Geometry: final body of the model. Coordinates: model frame, mm. Round coordinates to 2 decimals unless told otherwise and drop trailing zeros. Write each loop counter-clockwise with the first axis right and the second up, starting at its lowest first coordinate (ties: lowest second). Pieces come first, ordered by that corner, then holes. Notation, with made-up numbers: M 63,58.25 L 81,58.25 A13 ccw 81,78.25 Z; hole C 51.5,-39 d5. An arc over 180 degrees is marked long. Answer as CSV lines item,"result". Start each with the question number.
Q1. Section query C-C on y = 3. Output: boundary loops of the cut face in (x, z).
Q2. Ray query, probe 1 along X at (y, z) = (0.85, 22.5); probe 2 along Z at (x, y) = (-14, 3.5); probe 3 along Z at (x, y) = (-14, 1). Return the intervals inside material, ascending.
Q3. First-contact query: pin 1 (1 mm diameter, centred on y = 0.5, z = 13.5, fed in from -X); pin 2 (1.5 mm diameter, centred on x = -42, y = 1, fed in from +Z); pin 3 (2 mm diameter, centred on y = 1, z = 15, fed in from +X). Flat tips, straight axial feed; report the tip coordinate or a pass-through.
```python
from build123d import *

# Parameters (mm, degrees)
SKETCH1_W           = 200
SKETCH1_H           = 80
BOSS_EXTRUDE1_DEPTH = 2
SKETCH2_W           = 196
SKETCH2_H           = 76
BOSS_EXTRUDE2_DEPTH = 2
FILLET1_R           = 2
FILLET2_R           = 2
FILLET3_R           = 2
SKETCH3_R           = 33.072163117
CUT_EXTRUDE1_DEPTH  = 25
FILLET4_R           = 2
FILLET5_R           = 2
SKETCH4_W           = 18.581197799
SKETCH4_H           = 6.58
CUT_EXTRUDE3_DEPTH  = 2
SKETCH5_W           = 3.741738876
SKETCH5_H           = 6.58
CUT_EXTRUDE4_DEPTH  = 2
FILLET6_R           = 2
FILLET7_R           = 2


with BuildPart() as part:
    # Sketch1 → Boss-Extrude1 (new body)
    with BuildSketch(Plane(origin=(0, 0, 0), x_dir=(1, 0, 0), z_dir=(0, 1, 0))):
        Rectangle(SKETCH1_W, SKETCH1_H)
    extrude(amount=BOSS_EXTRUDE1_DEPTH)

    # Sketch2 → Boss-Extrude2 (add)
    with BuildSketch(Plane(origin=(0, 2, 0), x_dir=(1, 0, 0), z_dir=(0, 1, 0))):
        Rectangle(SKETCH2_W, SKETCH2_H)
    extrude(amount=BOSS_EXTRUDE2_DEPTH)

    # Fillet1
    fillet1_edges = [part.edges().sort_by_distance(p)[0] for p in [
        (-100, 1, -40),
        (100, 1, -40),
        (100, 1, 40),
        (-100, 1, 40),
    ]]
    fillet(fillet1_edges, radius=FILLET1_R)

    # Fillet2
    fillet2_edges = [part.edges().sort_by_distance(p)[0] for p in [
        (-98, 3, -38),
        (-98, 3, 38),
        (98, 3, 38),
        (98, 3, -38),
    ]]
    fillet(fillet2_edges, radius=FILLET2_R)

    # Fillet3
    fillet3_edges = [part.edges().sort_by_distance(p)[0] for p in [
        (-99.414213562, 0, -39.414213562),
        (0, 0, -40),
        (99.414213562, 0, -39.414213562),
        (100, 0, 0),
        (99.414213562, 0, 39.414213562),
        (0, 0, 40),
        (-99.414213562, 0, 39.414213562),
        (-97.414213562, 2, 37.414213562),
        (-98, 2, 0),
        (-97.414213562, 2, -37.414213562),
        (0, 2, -38),
        (97.414213562, 2, -37.414213562),
        (98, 2, 0),
        (97.414213562, 2, 37.414213562),
        (-100, 0, 0),
        (0, 2, 38),
    ]]
    fillet(fillet3_edges, radius=FILLET3_R - 0.0001)  # a hair under: the kernel refuses the full size

    # Sketch3 → Cut-Extrude1 (cut)
    with BuildSketch(Plane.XZ):
        with Locations(Location((-43.56, 0, 0), (0, 0, 270))):
            Circle(SKETCH3_R)
    extrude(amount=-CUT_EXTRUDE1_DEPTH, mode=Mode.SUBTRACT)

    # Fillet4
    fillet4_edges = [part.edges().sort_by_distance(p)[0] for p in [
        (-43.56, 0, 33.072163117),
    ]]
    fillet(fillet4_edges, radius=FILLET4_R)

    # Fillet5
    fillet5_edges = [part.edges().sort_by_distance(p)[0] for p in [
        (-43.56, 4, 33.072163117),
    ]]
    fillet(fillet5_edges, radius=FILLET5_R - 0.0001)  # a hair under: the kernel refuses the full size

    # Sketch4 → Cut-Extrude3 (cut)
    with BuildSketch(Plane(origin=(0, 4, 0), x_dir=(1, 0, 0), z_dir=(0, 1, 0))):
        with Locations((88.709401101, 20.450898194)):
            Rectangle(SKETCH4_W, SKETCH4_H)
    extrude(amount=-CUT_EXTRUDE3_DEPTH, mode=Mode.SUBTRACT)

    # Sketch5 → Cut-Extrude4 (cut)
    with BuildSketch(Plane(origin=(0, 2, 0), x_dir=(1, 0, 0), z_dir=(0, 1, 0))):
        with Locations((99.870869438, 20.450898194)):
            Rectangle(SKETCH5_W, SKETCH5_H)
    extrude(amount=CUT_EXTRUDE4_DEPTH, mode=Mode.SUBTRACT)

    # Fillet6
    fillet6_edges = [part.edges().sort_by_distance(p)[0] for p in [
        (79.418802201, 3, -17.160898194),
        (79.418802201, 3, -23.740898194),
    ]]
    fillet(fillet6_edges, radius=FILLET6_R)

    # Fillet7
    fillet7_edges = [part.edges().sort_by_distance(p)[0] for p in [
        (80.004588639, 4, -17.746684631),
        (80.004588639, 4, -23.155111756),
        (79.418802201, 4, -20.450898194),
        (89.709401101, 4, -17.160898194),
        (89.709401101, 4, -23.740898194),
    ]]
    fillet(fillet7_edges, radius=FILLET7_R - 0.0001)  # a hair under: the kernel refuses the full size


solid = part.part
```
Entries:
1,outline,"M -98.27,-36 A2.27 ccw -96,-38.27 L 96,-38.27 A2.27 ccw 98.27,-36 L 98.27,-24.01 L 81.42,-24.01 A2.27 cw 79.15,-21.74 L 79.15,-19.16 A2.27 cw 81.42,-16.89 L 98.27,-16.89 L 98.27,36 A2.27 ccw 96,38.27 L -96,38.27 A2.27 ccw -98.27,36 Z; hole C -43.56,0 d66.68"
2,probe 1,"x = -99.64 to -68.29, -18.83 to 99.64"
2,probe 2,"z = -38.06 to -16.29, 16.29 to 38.06"
2,probe 3,"z = -39.73 to -15.42, 15.42 to 39.73"
3,pin 1,"stops at x = -99.73"
3,pin 2,"stops at z = 39.98"
3,pin 3,"stops at x = 100"
